Here's how the part is built. I have some questions about the finished solid (model axes, mm). Face numbers are marked on the shaded views. A direction names the side the tool comes from. Coordinates: 2 decimals unless noted, no trailing zeros. Write each loop counter-clockwise with the first axis right and the second up, starting at its lowest first coordinate (ties: lowest second). Pieces come first, ordered by that corner, then holes. Notation, with made-up numbers: (13, 54) - (25, 54) arc R14 cw to (25, 72) - close; hole circle Ø2 at (5, 76). An arc over 180 degrees is marked (long way). Answer in a Markdown table with one row per item. Add a question column.
Item 1: If I drill on probe 1 along Z at (x, y) = (0, 2); probe 2 along Y at (x, z) = (42, 9); probe 3 along X at (y, z) = (44, -1), over which ranges is the centre line in solid material (lowest first)? Write a range as from..to.
Item 2: I'm going to push flat-ended pins straight in: pin 1 (3 mm diameter, centred on x = 11.5, y = 62.5, fed in from -Z); pin 2 (1 mm diameter, centred on x = 12, y = 68, fed in from +Z); pin 3 (3 mm diameter, centred on x = 12.5, y = 58, fed in from +Z). Where does each tip first touch, or does it pass through?
Item 3: Imagine slicing it at A-A (z = 0). State how many separate pieces and enclosed holes the cut face has, plus the area to 3 significant figures.
Item 4: Imagine slicing it at C-C (z = 26). Please give me the cut outline in (x, y), plus the area to 3 significant figures.
Item 5: We'd pull the mould along Y, two halves only. Please class the marked faces 1, 2 and 3: +Y half, -Y half, draft (parallel to the pull), parting line (faces both ways), or undercut.
Item 6: Imagine slicing it at D-D (y = 52). Please give me the cut outline in (x, z).
Item 7: Which directions (+Z, -Z, +X, -X, +Y, -Y) give clear straight access to the entire face, cutting with the end or side of a thin tool? Please do the marked faces 4 and 5.
from build123d import *

# Parameters (mm, degrees)
M3_CLEARANCE_HOLE1_D     = 3.4
M3_CLEARANCE_HOLE1_DEPTH = 4.001
M3_CLEARANCE_HOLE2_D     = 3.4
M3_CLEARANCE_HOLE2_DEPTH = 4.001
CIRPATTERN1_COUNT        = 12


with BuildPart() as part:
    # Sketch1 → Revolve1 (revolve)
    with BuildSketch(Plane.XY):
        Polygon((-32, 83.984026871), (-32, 0), (-46, 0), (-46, 4), (-36, 4), (-36, 79.984026871), (-46, 79.984026871), (-46, 83.984026871), align=None)
    revolve(axis=Axis((0, 0, 0), (0, 1, 0)))

    # M3 Clearance Hole1
    with Locations(Plane(origin=(0, 83.984026871, 0), x_dir=(1, 0, 0), z_dir=(0, 1, 0))):
        with Locations((0, 41)):
            m3_clearance_hole1 = Hole(M3_CLEARANCE_HOLE1_D / 2, depth=M3_CLEARANCE_HOLE1_DEPTH)

    # M3 Clearance Hole2
    with Locations(Plane(origin=(0, 0, 0), x_dir=(-1, 0, 0), z_dir=(0, -1, 0))):
        with Locations((0, 41)):
            m3_clearance_hole2 = Hole(M3_CLEARANCE_HOLE2_D / 2, depth=M3_CLEARANCE_HOLE2_DEPTH)

    # CirPattern1: M3 Clearance Hole1, M3 Clearance Hole2 ×12 about axis
    cirpattern1_axis = Axis((0, 0, 0), (0, 1, 0))
    for i in range(1, CIRPATTERN1_COUNT):
        add(m3_clearance_hole1.rotate(cirpattern1_axis, i * 360 / CIRPATTERN1_COUNT), mode=Mode.SUBTRACT)
        add(m3_clearance_hole2.rotate(cirpattern1_axis, i * 360 / CIRPATTERN1_COUNT), mode=Mode.SUBTRACT)


solid = part.part
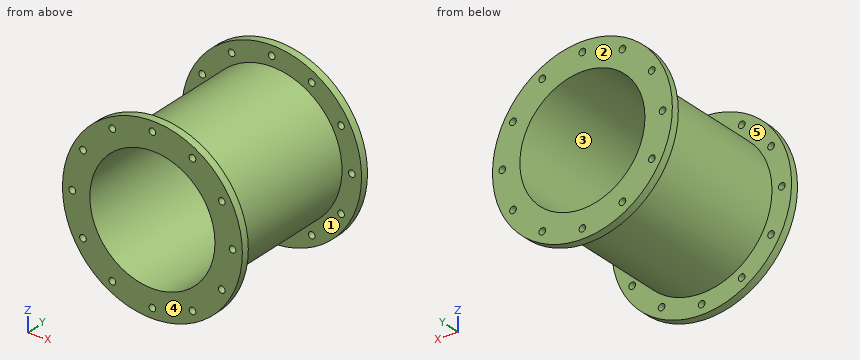
Here are the results:
| question | item | result |
|---|---|---|
| 1 | probe 1 | z = -46..-42.7, -39.3..-32, 32..39.3, 42.7..46 |
| 1 | probe 2 | y = 0..4, 79.98..83.98 |
| 1 | probe 3 | x = -35.99..-31.98, 31.98..35.99 |
| 2 | pin 1 | stops at z = -34.58 |
| 2 | pin 2 | stops at z = 34.11 |
| 2 | pin 3 | stops at z = 34.28 |
| 3 | separate pieces | 6 |
| 3 | enclosed holes | 0 |
| 3 | area | 777 mm2 |
| 4 | outline | (-37.95, 0) - (-18.65, 0) - (-18.65, 83.98) - (-37.95, 83.98) - (-37.95, 79.98) - (-24.9, 79.98) - (-24.9, 4) - (-37.95, 4) - close; (18.65, 0) - (37.95, 0) - (37.95, 4) - (24.9, 4) - (24.9, 79.98) - (37.95, 79.98) - (37.95, 83.98) - (18.65, 83.98) - close |
| 4 | area | 1,260 mm2 |
| 5 | face 1 | undercut |
| 5 | face 2 | +Y half |
| 5 | face 3 | draft |
| 6 | outline | circle Ø72 at (0, 0); hole circle Ø64 at (0, 0) |
| 7 | face 4 | +Z, -Z, +X, -X, -Y |
| 7 | face 5 | none |
